The figure shows three views and two pictorial views of one solid part (mm, origin at its lowest corner). Answer the questions. Round coordinates to 2 decimals unless told otherwise and drop trailing zeros. Order: outer loops, then holes, each group sorted by start corner. A loop starts at its lowest first (then second) coordinate and runs counter-clockwise, first axis right, second up. Notation, with made-up numbers: (33, -2.75) - (62, -2.75) arc R11 ccw to (62, 18.25) - close; hole circle Ø5 at (47, -15.75). An arc over 180 degrees is marked (long way). Answer in a Markdown table with one row per item.
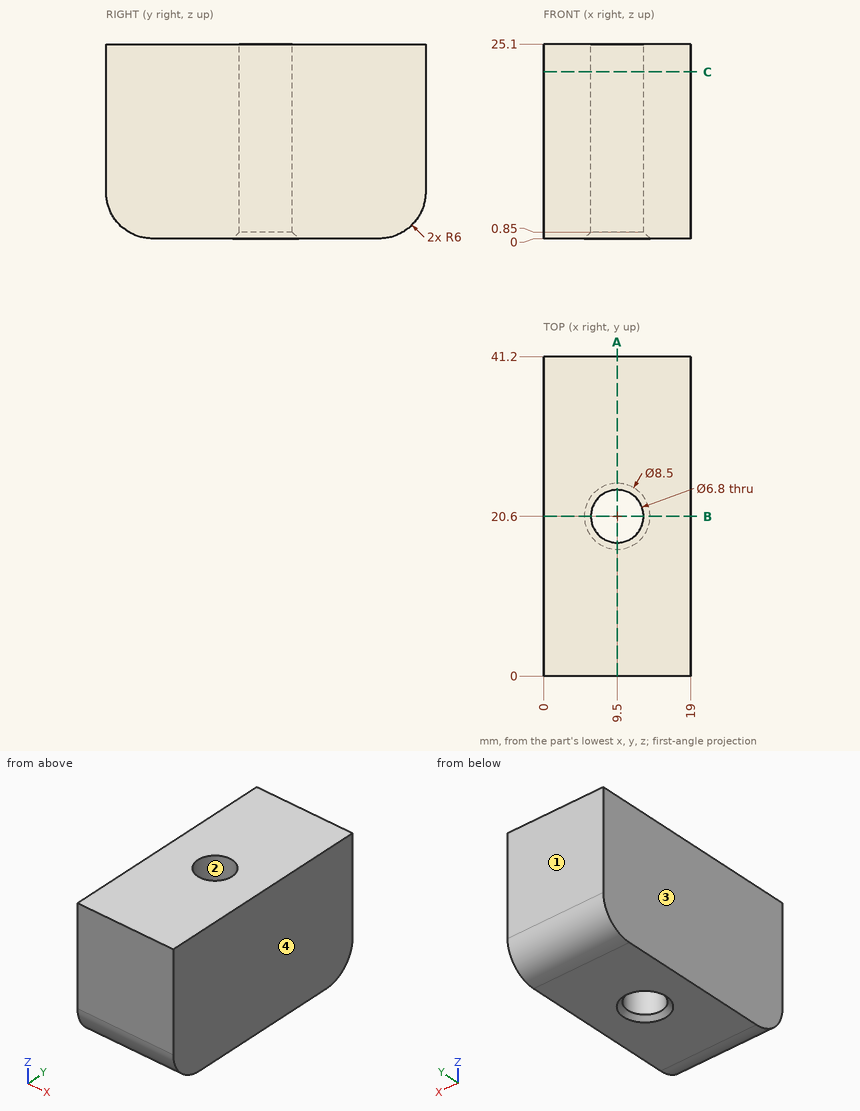
1) Find section C-C, the plane z = 21.5. Give the vertices of the cut face in (x, y), then the cut area to 3 significant figures.
Filled in:
| item | result |
|---|---|
| outline | (0, 0) - (19, 0) - (19, 41.2) - (0, 41.2) - close; hole circle Ø6.8 at (9.5, 20.6) |
| area | 746 mm^2 |
2) Find section B-B, the plane y = 20.6. Give the vertices of the cut face in (x, z), then the cut area to 3 significant figures.
Filled in:
| item | result |
|---|---|
| outline | (0, 0) - (5.25, 0) - (6.1, 0.85) - (6.1, 25.1) - (0, 25.1) - close; (12.9, 0.85) - (13.75, 0) - (19, 0) - (19, 25.1) - (12.9, 25.1) - close |
| area | 305 mm^2 |
3) The mould has two halves that part along X. Classify the marked faces 1, 2, 3 and 4: released by +X, released by -X, zero draft, split by the parting line, or undercut.
Filled in:
| item | result |
|---|---|
| face 1 | zero draft |
| face 2 | undercut |
| face 3 | released by -X |
| face 4 | released by +X |
4) Find the intervals of material crossed by probe 1 along Y at (x, z) = (9.5, 8.5); probe 2 along X at (y, z) = (18, 21.5); probe 3 along X at (y, z) = (20.6, 19.25), in increasing order. Write a range as from..to.
Filled in:
| item | result |
|---|---|
| probe 1 | y = 0..17.2, 24..41.2 |
| probe 2 | x = 0..7.31, 11.69..19 |
| probe 3 | x = 0..6.1, 12.9..19 |
5) Find section A-A, the plane x = 9.5. Give the vertices of the cut face in (y, z).
Filled in:
| item | result |
|---|---|
| outline | (0, 6) arc R6 ccw to (6, 0) - (16.35, 0) - (17.2, 0.85) - (17.2, 25.1) - (0, 25.1) - close; (24, 0.85) - (24.85, 0) - (35.2, 0) arc R6 ccw to (41.2, 6) - (41.2, 25.1) - (24, 25.1) - close |
6) Each of these flat-tipped pins is pushed along its axis until it touches: pin 1 (6 mm diameter, centred on x = 9.5, y = 20.6, fed in from -Z); pin 2 (12 mm diameter, centred on y = 8, z = 21.5, fed in from -X). Where does it stop, or does it pass through?
Filled in:
| item | result |
|---|---|
| pin 1 | passes through |
| pin 2 | stops at x = 0 |
